CAD build for the part. Positions are in the model's coordinates, mm. A direction names the side the tool comes from. Coordinates: 2 decimals unless noted, no trailing zeros. Order: outer loops, then holes, each group sorted by start corner. A loop starts at its lowest first (then second) coordinate and runs counter-clockwise, first axis right, second up. Notation, with made-up numbers: (19, 59) - (65, 59) arc R29 cw to (65, 98) - close; hole circle Ø3 at (49.5, -1.5). An arc over 180 degrees is marked (long way). Return JSON: item names as keys, results as strings.
from build123d import *

# Parameters (mm, degrees)
SKETCH1_W          = 19.05
SKETCH1_H          = 25.4
MAIN_BODY_DEPTH    = 25.4
HOLLOW_IT_T        = -2.54
SKETCH3_R          = 3.81
NIBBLE_NO_1_DEPTH  = 12.7
NIBBLE_START       = 12.7
SKETCH4_R          = 3.81
NIBBLE_NO_2_DEPTH  = 12.7
SKETCH5_W          = 1.27
SKETCH5_H          = 3.81
FLAG_DEPTH         = 0.254
SKETCH2_R          = 3.81
NIBBLE_HOLES_DEPTH = 45.45
SMOOTHNESS_R       = 2.54


with BuildPart() as part:
    # Sketch1 → main body (new body)
    with BuildSketch(Plane.XY):
        Rectangle(SKETCH1_W, SKETCH1_H)
    extrude(amount=MAIN_BODY_DEPTH)

    # hollow it
    hollow_it_openings = [part.faces().sort_by_distance(p)[0] for p in [
        (0, 12.7, 12.7),
    ]]
    offset(amount=HOLLOW_IT_T, openings=hollow_it_openings, kind=Kind.INTERSECTION)

    # Sketch3 → nibble no 1 (add)
    with BuildSketch(Plane.XY.offset(25.4)):
        with Locations(Location((0, 0, 0), (0, 0, 180))):
            Circle(SKETCH3_R)
    extrude(amount=NIBBLE_NO_1_DEPTH)

    # Sketch4 → nibble no 2 (add)
    with BuildSketch(Plane(origin=(0, 0, 0), x_dir=(-1, 0, 0), z_dir=(0, 0, -1)).offset(NIBBLE_START)):
        Circle(SKETCH4_R)
    extrude(amount=-NIBBLE_NO_2_DEPTH)

    # Sketch5 → flag (add)
    with BuildSketch(Plane(origin=(0, 0, 0), x_dir=(-1, 0, 0), z_dir=(0, -1, 0))):
        with Locations((-0.18666561, 6.353298227)):
            Rectangle(SKETCH5_W, SKETCH5_H)
    extrude(amount=FLAG_DEPTH)

    # Sketch2 → nibble holes (cut, through all)
    with BuildSketch(Plane(origin=(9.525, 0, 0), x_dir=(0, 0, -1), z_dir=(1, 0, 0))):
        with Locations((-12.7, 0)):
            Circle(SKETCH2_R)
    extrude(amount=-NIBBLE_HOLES_DEPTH, mode=Mode.SUBTRACT)

    # smoothness
    smoothness_edges = [part.edges().sort_by_distance(p)[0] for p in [
        (0, -12.7, 25.4),
        (6.985, -10.16, 12.7),
        (0, 12.7, 2.54),
        (6.985, 12.7, 12.7),
        (-6.985, 12.7, 12.7),
        (0, -10.16, 2.54),
        (-6.985, -10.16, 12.7),
        (0, 12.7, 22.86),
        (0, -10.16, 22.86),
        (3.81, 0, 25.4),
        (3.81, 0, 38.1),
        (3.81, 0, 0),
        (3.81, 0, -12.7),
        (0, -12.7, 0),
        (9.525, -12.7, 12.7),
        (-9.525, -12.7, 12.7),
    ]]
    fillet(smoothness_edges, radius=SMOOTHNESS_R - 0.0001)  # a hair under: the kernel refuses the full size


solid = part.part
Item 1: Wall check: L1, parallel to Z at x = 3, y = 7.75; L2, parallel to X at y = -1.25, z = 4 (3 decimals); L3, parallel to Z at x = -7.75, y = 6. Give the ranges that are in metal, low to high. Write a range as [from, to].
Findings below:
{"L1": "z = [0, 2.54], [22.86, 25.4]", "L2": "x = [-9.525, -6.985], [6.985, 9.525]", "L3": "z = [0, 25.4]"}
Item 2: Band-saw the part on A-A, the plane z = 12.7. Count the separate pieces of the cut face and the enclosed holes in it, then the cut area to 3 significant figures.
Findings below:
{"separate pieces": "3", "enclosed holes": "0", "area": "123 mm²"}
Item 3: Mould opens along X. For faces 3 (the cylindrical face through (0.133, 11.976, 1.776)), 4 (the flat face through (-9.525, 4, 15)), 5 (the cylindrical face through (-6.261, -9.396, 12.558)), 6 (the flat face through (0, 7, 25.4)) say: released by +X, released by -X, zero draft, split by the parting line, or undercut.
Findings below:
{"face 3": "undercut", "face 4": "released by -X", "face 5": "undercut", "face 6": "zero draft"}
Item 4: Band-saw the part on B-B, the plane y = -7. List the corners of the cut face in (x, z) (3 decimals), then the cut area to 3 significant figures.
Findings below:
{"outline": "(-9.525, 0) - (9.525, 0) - (9.525, 25.4) - (-9.525, 25.4) - close; hole (-6.985, 2.54) - (6.985, 2.54) - (6.985, 22.86) - (-6.985, 22.86) - close", "area": "200 mm²"}
Item 5: Which spindle directions (+Z, -Z, +X, -X, +Y, -Y) get a long thin tool onto all of the face, cutting with end or side? Do faces 1 (the cylindrical face through (0.133, -11.976, 0.764)), 2 (the flat face through (0, -10.16, 13)). Say none if no direction does.
Findings below:
{"face 1": "-Z, +X, -X, -Y", "face 2": "+Y"}
Item 6: Drop flat-ended pins along their axis: P1, Ø10, axis at x = 1, z = 14.5, coming from the +Y side; P2, Ø4, axis at x = 3, y = 3, coming from the -Z side; P3, Ø8, axis at x = -4, z = 28, coming from the -Y side. Give the stop position or say it passes through.
Findings below:
{"P1": "stops at y = -9.63", "P2": "stops at z = -12.51", "P3": "stops at y = -12.43"}
